Autodesk Inventor part; units mm, degrees
ref_plane "YZ Plane" through (0, 0, 0) normal (1, 0, 0) x (0, 1, 0)
ref_plane "XZ Plane" through (0, 0, 0) normal (0, 1, 0) x (-1, 0, 0)
ref_plane "XY Plane" through (0, 0, 0) normal (0, 0, 1) x (1, 0, 0)
sketch "Schizzo1" plane through (0, 0, 0) normal (0, 0, 1) x (1, 0, 0)
  line L0 (-152.5, 86) -> (-2.5, 86) construction
  line L1 (-152.5, 0) -> (-152.5, 86) construction
  line L2 (-2.5, 0) -> (-2.5, 86) construction
  circle A0 centre (-9.5, 81) radius 1.5
  circle A1 centre (-147.5, 81) radius 1.5
  circle A2 centre (-147.5, 17) radius 1.5
  line L3 (4, 95) -> (-161, 95)
  line L4 (-161, -24) -> (-133, -24)
  line L5 (-128, -19) -> (-128, -19)
  line L6 (-123, -14) -> (-100, -14)
  line L7 (-95, -19) -> (-95, -19)
  line L8 (-90, -24) -> (-67, -24)
  line L9 (-62, -19) -> (-62, -19)
  line L10 (-57, -14) -> (-34, -14)
  line L11 (-29, -19) -> (-29, -19)
  line L12 (-24, -24) -> (4, -24)
  arc A3 (-133, -24) -> (-128, -19) centre (-133, -19) ccw
  arc A4 (-123, -14) -> (-128, -19) centre (-123, -19) ccw
  arc A5 (-95, -19) -> (-100, -14) centre (-100, -19) ccw
  arc A6 (-95, -19) -> (-90, -24) centre (-90, -19) ccw
  arc A7 (-67, -24) -> (-62, -19) centre (-67, -19) ccw
  arc A8 (-57, -14) -> (-62, -19) centre (-57, -19) ccw
  arc A9 (-29, -19) -> (-34, -14) centre (-34, -19) ccw
  arc A10 (-29, -19) -> (-24, -24) centre (-24, -19) ccw
  arc A11 (-17, 81) -> (-9.5, 73.5) centre (-9.5, 81) ccw
  arc A12 (-147.5, 73.5) -> (-140, 81) centre (-147.5, 81) ccw
  arc A13 (-140.4901, 19.6667) -> (-147.5, 24.5) centre (-147.5, 17) ccw
  line L13 (-147.5, 73.5) -> (-147.5, 24.5)
  line L14 (-17, 81) -> (-140, 81)
  line L15 (-9.5, 10) -> (-126.4703, 10)
  arc A14 (-140.4901, 19.6667) -> (-126.4703, 10) centre (-126.4703, 25) ccw
  line L16 (-9.5, 10) -> (-9.5, 73.5)
  line L17 (-161, 95) -> (-161, -24)
  line L18 (4, 95) -> (4, -24)
  line L19 (-161, -4) -> (-150, -4)
  line L20 (-150, 0) -> (-150, -4)
  line L21 (-150, 0) -> (-161, 0)
  line L22 (-161, 0) -> (-161, -4)
  line L23 (-139, -4) -> (-128, -4)
  line L24 (-128, 0) -> (-128, -4)
  line L25 (-128, 0) -> (-139, 0)
  line L26 (-139, 0) -> (-139, -4)
  line L27 (-117, -4) -> (-106, -4)
  line L28 (-106, 0) -> (-106, -4)
  line L29 (-106, 0) -> (-117, 0)
  line L30 (-117, 0) -> (-117, -4)
  line L31 (-95, -4) -> (-84, -4)
  line L32 (-84, 0) -> (-84, -4)
  line L33 (-84, 0) -> (-95, 0)
  line L34 (-95, 0) -> (-95, -4)
  line L35 (-73, -4) -> (-62, -4)
  line L36 (-62, 0) -> (-62, -4)
  line L37 (-62, 0) -> (-73, 0)
  line L38 (-73, 0) -> (-73, -4)
  line L39 (-51, -4) -> (-40, -4)
  line L40 (-40, 0) -> (-40, -4)
  line L41 (-40, 0) -> (-51, 0)
  line L42 (-51, 0) -> (-51, -4)
  line L43 (-29, -4) -> (-18, -4)
  line L44 (-18, 0) -> (-18, -4)
  line L45 (-18, 0) -> (-29, 0)
  line L46 (-29, 0) -> (-29, -4)
  line L47 (-7, -4) -> (4, -4)
  line L48 (-7, 0) -> (-7, -4)
  line L49 (-147.5, 82.5) -> (-147.5, 79.5) construction
  line L50 (-149, 82.5) -> (-149, 79.5)
  line L51 (-146, 79.5) -> (-146, 82.5)
  arc A15 (-146, 82.5) -> (-149, 82.5) centre (-147.5, 82.5) ccw
  arc A16 (-149, 79.5) -> (-146, 79.5) centre (-147.5, 79.5) ccw
  line L52 (-9.5, 82.5) -> (-9.5, 79.5) construction
  line L53 (-11, 82.5) -> (-11, 79.5)
  line L54 (-8, 79.5) -> (-8, 82.5)
  arc A17 (-8, 82.5) -> (-11, 82.5) centre (-9.5, 82.5) ccw
  arc A18 (-11, 79.5) -> (-8, 79.5) centre (-9.5, 79.5) ccw
  line L55 (-147.5, 18.5) -> (-147.5, 15.5) construction
  line L56 (-149, 18.5) -> (-149, 15.5)
  line L57 (-146, 15.5) -> (-146, 18.5)
  arc A19 (-146, 18.5) -> (-149, 18.5) centre (-147.5, 18.5) ccw
  arc A20 (-149, 15.5) -> (-146, 15.5) centre (-147.5, 15.5) ccw
  line L58 (4, 0) -> (4, -4)
  line L59 (4, 0) -> (-7, 0)
  point P0 (-128, -24)
  point P1 (-128, -14)
  point P2 (-95, -14)
  point P3 (-95, -24)
  point P4 (-62, -24)
  point P5 (-62, -14)
  point P6 (-29, -14)
  point P7 (-29, -24)
  point P8 (-144.8074, 10)
  dimension "d0" = 165
  dimension "d9" = 33
  dimension "d10" = 10
  dimension "d11" = 33
  dimension "d12" = 10
  dimension "d13" = 33
  dimension "d14" = 10
  dimension "d15" = 33
  dimension "d16" = 5
  dimension "d21" = 15
extrude "Estrusione1" add sketch "Schizzo1" along normal blind 4 contours L18 L59 L48 L47 L12 A10 A9 L10 A8 A7 L8 A6 A5 L6 A4 A3 L4 L17 L19 L20 L21 L3
sketch "Schizzo2" plane through (0, 0, 4) normal (0, 0, 1) x (1, 0, 0)
  line L0 (-157, 85.5) -> (-161, 85.5)
  line L1 (-161, 85.5) -> (-161, 95)
  line L2 (-161, 95) -> (-157, 95)
  line L3 (-157, 95) -> (-157, 85.5)
  line L4 (-157, 66.5) -> (-161, 66.5)
  line L5 (-161, 66.5) -> (-161, 76)
  line L6 (-161, 76) -> (-157, 76)
  line L7 (-157, 76) -> (-157, 66.5)
  line L8 (-161, 57) -> (-157, 57)
  line L9 (-157, 57) -> (-157, 47.5)
  line L10 (-157, 47.5) -> (-161, 47.5)
  line L11 (-161, 47.5) -> (-161, 57)
  line L12 (-157, 28.5) -> (-161, 28.5)
  line L13 (-161, 28.5) -> (-161, 38)
  line L14 (-161, 38) -> (-157, 38)
  line L15 (-157, 38) -> (-157, 28.5)
  line L16 (-161, 19) -> (-157, 19)
  line L17 (-157, 19) -> (-157, 9.5)
  line L18 (-157, 9.5) -> (-161, 9.5)
  line L19 (-161, 9.5) -> (-161, 19)
  point P0 (0, 0)
extrude "Estrusione2" cut sketch "Schizzo2" against normal blind 4
fillet "Raccordo1" radius 15 1 edges at (4, 95, 2)
fillet "Raccordo2" radius 10 1 edges at (4, -24, 2)
sketch "Schizzo3" plane through (0, 0, 4) normal (0, 0, 1) x (1, 0, 0)
  line L0 (-14.15, 0) -> (-10.85, 0)
  line L1 (-146.15, 0) -> (-142.85, 0)
  line L2 (-144.5, 0) -> (-137.5, 0) construction
  line L3 (-12.5, 0) -> (-12.5, -17) construction
  circle A0 centre (-12.5, -17) radius 1.65
  line L4 (-157, 82.4) -> (-157, 79.1) construction
  line L5 (-157, 85.5) -> (-157, 95) construction
  line L6 (-157, 95) -> (-157, 85.5)
  line L7 (-157, 90.25) -> (-144, 90.25) construction
  circle A1 centre (-144, 90.25) radius 1.65
  line L8 (-157, -12.35) -> (-157, -15.65) construction
  line L9 (-157, -14) -> (-144, -14) construction
  circle A2 centre (-144, -14) radius 1.65
  point P0 (0, 0)
  dimension "d32" = 3.3
  dimension "d35" = 13
  dimension "d36" = 3.3
  dimension "d37" = 13
  dimension "d38" = 3.3
  dimension "d39" = 17
extrude "Estrusione3" cut sketch "Schizzo3" against normal blind 4
properties part number "LatoAlimentatore"
The model under review builds one solid part; all positions refer to its coordinate system, in mm. A direction names the side the tool comes from. Give positions to 0.01 mm unless a question says otherwise; leave off trailing zeros. Order: outer loops, then holes, each group sorted by start corner. A loop starts at its lowest first (then second) coordinate and runs counter-clockwise, first axis right, second up. Notation, with made-up numbers: M 67,-19.75 L 86,-19.75 A7 cw 86,-12.75 Z; hole C -19.5,-2.75 d7. An arc over 180 degrees is marked long. Answer in a Markdown table with one row per item. Add a question column.
1. Mouldability with a two-part tool opening along Y and no side actions: class faces 4 (the flat face through (-157, 33, 2)), 5 (the flat face through (-112, -14, 2)), 6 (the flat face through (-161, 62, 2)) as released by +Y, released by -Y, zero draft, split by the parting line, or undercut.
2. Add section C-C on z = 1.9. Count the separate pieces of the cut face and the enclosed holes in it, plus the area to 3 significant figures.
3. Add section A-A on x = -20.5. State the section outline as (y, z) points.
4. Add section D-D on y = 90.25. State the section outline as (x, z) points.
5. Machinability: for faces 1 (the flat face through (-159, 76, 2)), 2 (the flat face through (-161, 81, 2)), 3 (the flat face through (-67, 0, 2)), which of the approach directions +Z, -Z, +X, -X, +Y, -Y give a long, thin tool a straight path to every point of the face, cutting with its end or side? Answer none if there is none.
6. To check wall thickness, follow line 1 along Y through (x, z) = (-87, 3.7); line 2 along Y through (x, z) = (-51.5, 3.3); line 3 along Y through (x, z) = (-144, 3). State the ranges of each line that lie inside material, in increasing order.
7. For pin 1 Ø4 at (x, y) = (-144, 90.25) entering from -Z; pin 2 Ø1.5 at (y, z) = (-2, 3.5) entering from -X; pin 3 Ø1.2 at (y, z) = (-2.5, 2.5) entering from +X; pin 4 Ø1.5 at (x, z) = (-56.5, 2.5) entering from -Y, all flat-tipped, find the tip position at first contact; note any pin that passes through.
8. Add section B-B on y = 31. State the section outline as (x, z) points.
The answers:
| question | item | result |
|---|---|---|
| 1 | face 4 | undercut |
| 1 | face 5 | released by -Y |
| 1 | face 6 | zero draft |
| 2 | separate pieces | 1 |
| 2 | enclosed holes | 13 |
| 2 | area | 8,710 mm2 |
| 3 | outline | M -24,0 L -4,0 L -4,4 L -24,4 Z; M 0,0 L 10,0 L 10,4 L 0,4 Z; M 81,0 L 95,0 L 95,4 L 81,4 Z |
| 4 | outline | M -157,0 L -145.65,0 L -145.65,4 L -157,4 Z; M -142.35,0 L -0.05,0 L -0.05,4 L -142.35,4 Z |
| 5 | face 1 | +Z, -Z, -X |
| 5 | face 2 | +Z, -Z, -X, +Y, -Y |
| 5 | face 3 | +Z, -Z |
| 6 | line 1 | -24 to -4, 0 to 10, 81 to 95 |
| 6 | line 2 | -14 to 10, 81 to 95 |
| 6 | line 3 | -24 to -15.65, -12.35 to 23.63, 74.37 to 88.6, 91.9 to 95 |
| 7 | pin 1 | z = 0 |
| 7 | pin 2 | x = -150 |
| 7 | pin 3 | x = -7 |
| 7 | pin 4 | y = -14.01 |
| 8 | outline | M -157,0 L -147.5,0 L -147.5,4 L -157,4 Z; M -9.5,0 L 4,0 L 4,4 L -9.5,4 Z |
